Geometry check sheet. Reference: the model listing, model coordinates, mm. Give positions to 0.01 mm unless a question says otherwise; leave off trailing zeros. Order: outer loops, then holes, each group sorted by start corner. A loop starts at its lowest first (then second) coordinate and runs counter-clockwise, first axis right, second up. Notation, with made-up numbers: M 4.5,68 L 23.5,68 A16 ccw 23.5,93 Z; hole C 1,21 d3. An arc over 180 degrees is marked long. Put each result on its own line as item: value. Start each with the question number.
Q1. Go/stop test with flat-tipped pins: pin 1 (0.7 mm diameter, centred on y = 1, z = -19.5, fed in from +X); pin 2 (1.5 mm diameter, centred on x = -48, y = 2.5, fed in from +Z); pin 3 (2.5 mm diameter, centred on x = -8, z = -12, fed in from -Y); pin 4 (6 mm diameter, centred on x = -129.5, y = 4, fed in from +Z). Record where each tip stops, or that it passes through.
Q2. Section check C-C on x = -51. Record the cut outline in (y, z), then the cut area to 3 significant figures.
Q3. Section check D-D on y = 4. Record the cut outline in (x, z), then the cut area to 3 significant figures.
Q4. Section check B-B on z = -36. Record the cut outline in (x, y).
Q5. Section check A-A on x = -124.5. Record the cut outline in (y, z), then the cut area to 3 significant figures.
Q6. Material ranges on L1, parallel to X at y = 0.7, z = -66; L2, parallel to X at y = 0.75, z = -74; L3, parallel to Z at x = -8, y = 1.4, recorded low to high.
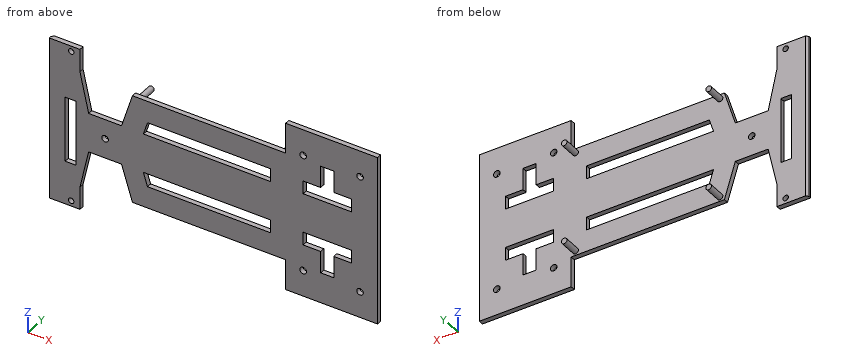
Autodesk Inventor part; units mm, degrees
ref_plane "YZ Plane" through (0, 0, 0) normal (1, 0, 0) x (0, 1, 0)
ref_plane "XZ Plane" through (0, 0, 0) normal (0, 1, 0) x (-1, 0, 0)
ref_plane "XY Plane" through (0, 0, 0) normal (0, 0, 1) x (1, 0, 0)
sketch "Sketch1" plane through (0, 0, 0) normal (0, 1, 0) x (-1, 0, 0)
  line L0 (42, -64) -> (112, -64)
  line L1 (112, -64) -> (112, -14)
  line L2 (112, -14) -> (42, -14)
  line L3 (112, -39) -> (112, -30)
  line L4 (112, -39) -> (112, -48)
  line L5 (112, -30) -> (136, -30)
  line L6 (136, -30) -> (136, -48)
  line L7 (136, -48) -> (112, -48)
  line L8 (112, -30) -> (117, -30)
  line L9 (117, -30) -> (112, -14)
  line L10 (112, -48) -> (117, -48)
  line L11 (117, -48) -> (112, -64)
  line L12 (136, -30) -> (136, -1.5)
  line L13 (136, -1.5) -> (150, -1.5)
  line L14 (136, -48) -> (136, -76.5)
  line L15 (136, -76.5) -> (150, -76.5)
  line L16 (150, -76.5) -> (150, -1.5)
  line L17 (42, -14) -> (42, 0)
  line L18 (42, 0) -> (42, -78)
  line L19 (42, -78) -> (0, -78)
  line L20 (0, -78) -> (0, 0)
  line L21 (0, 0) -> (42, 0)
  line L22 (136, -30) -> (132, -30)
  line L23 (136, -30) -> (136, -12)
  line L24 (136, -12) -> (132, -30)
  line L25 (136, -48) -> (132, -48)
  line L26 (136, -48) -> (136, -66)
  line L27 (136, -66) -> (132, -48)
  dimension "d3" = 70
  dimension "d4" = 50
  dimension "d5" = 9
  dimension "d6" = 9
  dimension "d7" = 24
  dimension "d8" = 18
  dimension "d9" = 5
  dimension "d10" = 5
  dimension "d11" = 28.5
  dimension "d12" = 14
  dimension "d13" = 28.5
  dimension "d14" = 14
  dimension "d20" = 78
  dimension "d21" = 42
  dimension "d22" = 14
  dimension "d23" = 14
  dimension "d24" = 1.5
  dimension "d25" = 94
  dimension "d26" = 4
  dimension "d27" = 18
  dimension "d28" = 4
  dimension "d29" = 18
extrude "Extrusion1" add sketch "Sketch1" along normal blind 2.2
sketch "Sketch2" plane through (0, 2.2, 0) normal (0, 1, 0) x (1, 0, 0)
  circle A0 centre (-34, 12) radius 1.5
  circle A1 centre (-8, 12) radius 1.5
  line L0 (-42, 0) -> (0, 0)
  line L1 (0, 0) -> (0, 78)
  line L2 (-42, 14) -> (-42, 0)
  circle A2 centre (-34, 66) radius 1.5
  circle A3 centre (-8, 66) radius 1.5
  line L3 (-42, 78) -> (-42, 64)
  line L4 (0, 78) -> (-42, 78)
  circle A4 centre (-124.5, 39) radius 1.5
  line L5 (-132, 30) -> (-117, 30)
  circle A5 centre (-140, 4) radius 1.25
  line L6 (-136, 1.5) -> (-136, 12)
  line L7 (-150, 1.5) -> (-136, 1.5)
  circle A6 centre (-140, 74) radius 1.25
  line L8 (-136, 66) -> (-136, 76.5)
  line L9 (-136, 76.5) -> (-150, 76.5)
  line L10 (-142.75, 26.5) -> (-137.75, 26.5)
  line L11 (-137.75, 26.5) -> (-137.75, 56.5)
  line L12 (-137.75, 56.5) -> (-142.75, 56.5)
  line L13 (-142.75, 56.5) -> (-142.75, 26.5)
  line L14 (-150, 76.5) -> (-150, 1.5)
  dimension "d32" = 3
  dimension "d33" = 3
  dimension "d34" = 12
  dimension "d35" = 8
  dimension "d36" = 8
  dimension "d37" = 12
  dimension "d38" = 3
  dimension "d39" = 3
  dimension "d40" = 8
  dimension "d41" = 12
  dimension "d42" = 12
  dimension "d43" = 8
  dimension "d44" = 9
  dimension "d45" = 7.5
  dimension "d46" = 3
  dimension "d47" = 2.5
  dimension "d48" = 4
  dimension "d49" = 2.5
  dimension "d50" = 2.5
  dimension "d51" = 4
  dimension "d52" = 2.5
  dimension "d53" = 5
  dimension "d54" = 30
  dimension "d55" = 20
  dimension "d56" = 7.25
extrude "Extrusion2" cut sketch "Sketch2" against normal blind 2.2
sketch "Sketch3" plane through (0, 2.2, 0) normal (0, 1, 0) x (1, 0, 0)
  line L0 (-42, 14) -> (-42, 0)
  line L1 (-42, 64) -> (-112, 64)
  line L2 (-42, 14) -> (-112, 14)
  line L3 (-112, 14) -> (-112, 64)
  line L4 (-112, 64) -> (-42, 64)
  line L5 (-42, 64) -> (-42, 14)
  circle A0 centre (-110, 16) radius 1.3
  circle A1 centre (-110, 62) radius 1.3
  circle A2 centre (-44, 16) radius 1.3
  circle A3 centre (-44, 62) radius 1.3
  point P0 (0, 0)
  dimension "d59" = 2
  dimension "d60" = 2
  dimension "d61" = 2.6
  dimension "d62" = 2
  dimension "d63" = 2
  dimension "d64" = 2.6
  dimension "d65" = 2.6
  dimension "d66" = 2.6
  dimension "d67" = 2
  dimension "d68" = 2
  dimension "d69" = 2
  dimension "d70" = 2
extrude "Extrusion3" add sketch "Sketch3" along normal blind 8 contours A0 | A1 | A2 | A3
sketch "Sketch4" plane through (0, 2.2, 0) normal (0, 1, 0) x (1, 0, 0)
  line L0 (-132, 30) -> (-117, 30)
  line L1 (-117, 30) -> (-112, 14)
  line L2 (-105.125, 24) -> (-107, 30)
  line L3 (-117, 48) -> (-132, 48)
  line L4 (-112, 64) -> (-117, 48)
  line L5 (-112, 64) -> (-102, 64)
  line L6 (-42, 64) -> (-112, 64)
  line L7 (-107, 48) -> (-105.125, 54)
  line L8 (-112, 14) -> (-42, 14)
  line L9 (-107, 30) -> (-49, 30)
  line L10 (-49, 30) -> (-49, 24)
  line L11 (-105.125, 24) -> (-49, 24)
  line L12 (-107, 48) -> (-49, 48)
  line L13 (-49, 48) -> (-49, 54)
  line L14 (-105.125, 54) -> (-49, 54)
  point P0 (0, 0)
  dimension "d79" = 10
  dimension "d88" = 10
  dimension "d93" = 10
  dimension "d111" = 58
  dimension "d112" = 6
  dimension "d113" = 10
  dimension "d114" = 6
  dimension "d115" = 72.646
  dimension "d116" = 58
  dimension "d117" = 56.125
  dimension "d118" = 18
  dimension "d119" = 6
  dimension "d120" = 6
extrude "Extrusion4" cut sketch "Sketch4" against normal blind 8
sketch "Sketch6" plane through (0, 2.2, 0) normal (0, 1, 0) x (1, 0, 0)
  line L0 (-34, 24) -> (-26, 24)
  line L1 (-26, 24) -> (-26, 14)
  line L2 (-26, 14) -> (-20, 14)
  line L3 (-34, 24) -> (-34, 30)
  line L4 (-34, 30) -> (-20, 30)
  line L5 (-20, 14) -> (-20, 24)
  line L6 (-20, 24) -> (-12, 24)
  line L7 (-12, 24) -> (-12, 30)
  line L8 (-12, 30) -> (-20, 30)
  line L9 (0, 0) -> (0, 78)
  line L10 (0, 39) -> (-41.084, 39)
  line L11 (-34, 54) -> (-26, 54)
  line L12 (-26, 54) -> (-26, 64)
  line L13 (-26, 64) -> (-20, 64)
  line L14 (-34, 54) -> (-34, 48)
  line L15 (-34, 48) -> (-20, 48)
  line L16 (-20, 64) -> (-20, 54)
  line L17 (-20, 54) -> (-12, 54)
  line L18 (-12, 54) -> (-12, 48)
  line L19 (-12, 48) -> (-20, 48)
  line L20 (-49, 30) -> (-49, 24)
  dimension "d97" = 8
  dimension "d98" = 10
  dimension "d99" = 6
  dimension "d100" = 16
  dimension "d101" = 6
  dimension "d102" = 10
  dimension "d103" = 8
  dimension "d104" = 6
  dimension "d105" = 9
  dimension "d121" = 15
extrude "Extrusion5" cut sketch "Sketch6" against normal blind 8
chamfer "Chamfer1" distance 1 angle 45 1 edges at (-150, 2.2, -39)
properties part number "onderplaat final"
Results found:
1. pin 1: stops at x = 0
1. pin 2: stops at z = -14
1. pin 3: passes through
1. pin 4: stops at z = -30
2. outline: M 0,-64 L 2.2,-64 L 2.2,-54 L 0,-54 Z; M 0,-48 L 2.2,-48 L 2.2,-30 L 0,-30 Z; M 0,-24 L 2.2,-24 L 2.2,-14 L 0,-14 Z
2. area: 83.6 mm^2
3. outline: C -110,-62 d2.6; C -110,-16 d2.6; C -44,-62 d2.6; C -44,-16 d2.6
3. area: 21.2 mm^2
4. outline: M -150,0 L -142.75,0 L -142.75,2.2 L -149,2.2 L -150,1.2 Z; M -137.75,0 L 0,0 L 0,2.2 L -137.75,2.2 Z
5. outline: M 0,-48 L 2.2,-48 L 2.2,-40.5 L 0,-40.5 Z; M 0,-37.5 L 2.2,-37.5 L 2.2,-30 L 0,-30 Z
5. area: 33.0 mm^2
6. L1: x = -150 to -136, -42 to -35.5, -32.5 to -9.5, -6.5 to 0
6. L2: x = -150 to -141.25, -138.75 to -136, -42 to 0
6. L3: z = -78 to -67.5, -64.5 to -13.5, -10.5 to 0
